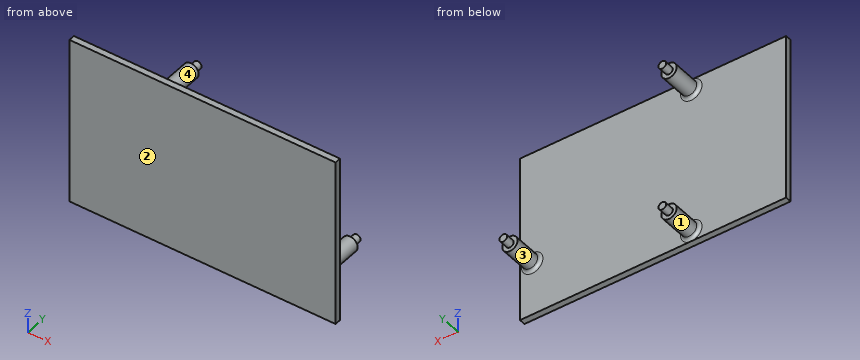
```python
from build123d import *

# Parameters (mm, degrees)
SKETCH1_W           = 87
SKETCH1_H           = 55
BOSS_EXTRUDE1_DEPTH = 2
SKETCH2_R           = 2.5
BOSS_EXTRUDE2_DEPTH = 10
SKETCH3_R           = 1.25
BOSS_EXTRUDE3_DEPTH = 3
FILLET2_R           = 1


with BuildPart() as part:
    # Sketch1 → Boss-Extrude1 (new body)
    with BuildSketch(Plane(origin=(0, 0, 0), x_dir=(1, 0, 0), z_dir=(0, 1, 0))):
        with Locations((43.5, 27.5)):
            Rectangle(SKETCH1_W, SKETCH1_H)
    extrude(amount=BOSS_EXTRUDE1_DEPTH)

    # Sketch2 → Boss-Extrude2 (add)
    with BuildSketch(Plane(origin=(0, 2, 0), x_dir=(1, 0, 0), z_dir=(0, 1, 0))):
        with Locations(Location((31, 51.5, 0), (0, 0, 90))):
            Circle(SKETCH2_R)
        with Locations(Location((31, 3.5, 0), (0, 0, 90))):
            Circle(SKETCH2_R)
        with Locations(Location((83, 37.5, 0), (0, 0, 90))):
            Circle(SKETCH2_R)
    extrude(amount=BOSS_EXTRUDE2_DEPTH)

    # Sketch3 → Boss-Extrude3 (add)
    with BuildSketch(Plane(origin=(0, 12, 0), x_dir=(1, 0, 0), z_dir=(0, 1, 0))):
        with Locations(Location((31, 51.5, 0), (0, 0, 270))):
            Circle(SKETCH3_R)
        with Locations(Location((31, 3.5, 0), (0, 0, 270))):
            Circle(SKETCH3_R)
        with Locations(Location((83, 37.5, 0), (0, 0, 270))):
            Circle(SKETCH3_R)
    extrude(amount=BOSS_EXTRUDE3_DEPTH)

    # Fillet2
    fillet2_edges = [part.edges().sort_by_distance(p)[0] for p in [
        (83, 2, -35),
        (31, 2, -1),
        (31, 2, -49),
    ]]
    fillet(fillet2_edges, radius=FILLET2_R - 0.0001)  # a hair under: the kernel refuses the full size


solid = part.part
```
Design review of the part built by this model. Coordinates are the model's own, in mm. Face numbers are marked on the shaded views. Coordinates: 2 decimals unless noted, no trailing zeros. Write each loop counter-clockwise with the first axis right and the second up, starting at its lowest first coordinate (ties: lowest second). Pieces come first, ordered by that corner, then holes.
1) Add section A-A (z = -3.5). Write out the cut boundary in (x, y).
2) Insertion check: pin 1 (5 mm diameter, centred on y = 11, z = -10, fed in from +X); pin 2 (6 mm diameter, centred on x = 37.5, z = -15.5, fed in from +Y); pin 3 (8 mm diameter, centred on y = 12.5, z = -37.5, fed in from +X). Each pin has a flat end and moves straight along its axis. Give the tip position at first contact, or say it passes through.
3) To check wall thickness, follow L1, parallel to Y at x = 54.5, z = -10.5; L2, parallel to Z at x = 29, y = 5.75; L3, parallel to Z at x = 32, y = 3.5. State the ranges of each line that lie inside material, in increasing order.
4) Add section B-B (x = 83). Write out the cut boundary in (y, z), plus the area to 3 significant figures.
5) Add section C-C (y = 7.5). Write out the cut boundary in (x, z), plus the area to 3 significant figures.
6) Mouldability with a two-part tool opening along Z and no side actions: class the marked faces 1, 2, 3 and 4 as +Z half, -Z half, draft (parallel to the pull), parting line (faces both ways), or undercut.
Check result:
1. outline: (0, 0) - (87, 0) - (87, 2) - (34.5, 2) arc R1 cw to (33.5, 3) - (33.5, 12) - (32.25, 12) - (32.25, 15) - (29.75, 15) - (29.75, 12) - (28.5, 12) - (28.5, 3) arc R1 cw to (27.5, 2) - (0, 2) - close
2. pin 1: passes through
2. pin 2: stops at y = 2
2. pin 3: stops at x = 85.5
3. L1: y = 0 to 2
3. L2: z = -53 to -50, -5 to -2
3. L3: z = -53.79 to -49.21, -5.79 to -1.21
4. outline: (0, -55) - (2, -55) - (2, -41) arc R1 cw to (3, -40) - (12, -40) - (12, -38.75) - (15, -38.75) - (15, -36.25) - (12, -36.25) - (12, -35) - (3, -35) arc R1 cw to (2, -34) - (2, 0) - (0, 0) - close
4. area: 168 mm2
5. outline: circle Ø5 at (31, -51.5); circle Ø5 at (31, -3.5); circle Ø5 at (83, -37.5)
5. area: 58.9 mm2
6. face 1: undercut
6. face 2: draft
6. face 3: parting line
6. face 4: undercut
